Read the model definition and answer for the solid it produces. Units are mm, in the model's axes. A direction names the side the tool comes from. Give positions to 0.01 mm unless a question says otherwise; leave off trailing zeros. Order: outer loops, then holes, each group sorted by start corner. A loop starts at its lowest first (then second) coordinate and runs counter-clockwise, first axis right, second up. Notation, with made-up numbers: M 31,85.25 L 40,85.25 A21 ccw 40,115.25 Z; hole C 82,-32.75 d6. An arc over 180 degrees is marked long. One line per item, written item: value.
from build123d import *

# Parameters (mm, degrees)
SKETCH2_R           = 17.5
BOSS_EXTRUDE2_DEPTH = 30
SKETCH3_R           = 11.5
CUT_EXTRUDE1_DEPTH  = 30
CUT_EXTRUDE1_DRAFT  = -5
SKETCH4_R           = 15
SKETCH4_R_2         = 12.5
CUT_EXTRUDE2_DEPTH  = 5
SKETCH8_R           = 11.5
BOSS_EXTRUDE3_DEPTH = 30
SWEEP3_PITCH        = 10.666666667
SWEEP3_HEIGHT       = 24
SWEEP3_RADIUS       = 7.5
SKETCH10_R          = 3.5
SKETCH11_R          = 5
BOSS_EXTRUDE4_DEPTH = 50
SKETCH16_R          = 3.036795298
CUT_EXTRUDE7_DEPTH  = 6


with BuildPart() as part:
    # Sketch2 → Boss-Extrude2 (new body)
    with BuildSketch(Plane(origin=(0, 0, 0), x_dir=(1, 0, 0), z_dir=(0, 1, 0))):
        with Locations(Location((0, 0, 0), (0, 0, 270))):
            Circle(SKETCH2_R)
    extrude(amount=BOSS_EXTRUDE2_DEPTH)


with BuildPart() as cut_extrude1_tool:
    # Sketch3 → Cut-Extrude1 (with draft: the straight prism first)
    with BuildSketch(Plane.XZ):
        Circle(SKETCH3_R)
    extrude(amount=-CUT_EXTRUDE1_DEPTH)
    # Cut-Extrude1: the draft: its side faces are tilted about the plane it starts from
    cut_extrude1_sides = [cut_extrude1_tool.faces().sort_by_distance(p)[0] for p in [
        (-11.5, 15, 0),
    ]]
    draft(cut_extrude1_sides, Plane.XZ, CUT_EXTRUDE1_DRAFT)


with BuildPart() as part_1:
    add(part.part)

    # Cut-Extrude1: cut by cut_extrude1_tool
    add(cut_extrude1_tool.part, mode=Mode.SUBTRACT)

    # Sketch4 → Cut-Extrude2 (cut)
    with BuildSketch(Plane.XZ):
        with Locations(Location((0, 0.439504446, 0), (0, 0, 270))):
            Circle(SKETCH4_R)
        with Locations(Location((0, 0.439504446, 0), (0, 0, 270))):
            Circle(SKETCH4_R_2, mode=Mode.SUBTRACT)
    extrude(amount=-CUT_EXTRUDE2_DEPTH, mode=Mode.SUBTRACT)


with BuildPart() as body_2:
    # Sketch8 → Boss-Extrude3 (new body)
    with BuildSketch(Plane.XZ):
        with Locations(Location((0, 0, 0), (0, 0, 270))):
            Circle(SKETCH8_R)
    extrude(amount=BOSS_EXTRUDE3_DEPTH)


with BuildPart() as body_3:
    # Sweep3: sweep along a helix
    with BuildLine() as sweep3_path:
        Helix(SWEEP3_PITCH, SWEEP3_HEIGHT, SWEEP3_RADIUS, center=(0, 0, 0), direction=(0, -1, 0), lefthand=True)
    # Sketch10 → Sweep3 (sweep)
    with BuildSketch(Plane(origin=(0, 0, 0), x_dir=(0, 0, -1), z_dir=(1, 0, 0))):
        with Locations((-7.5, -16)):
            Circle(SKETCH10_R)
    sweep(path=sweep3_path.line, is_frenet=True)


with BuildPart() as body_2_1:
    add(body_2.part)

    # Combine1: cut body 3
    add(body_3.part, mode=Mode.SUBTRACT)

    # Sketch11 → Boss-Extrude4 (add)
    with BuildSketch(Plane.XZ.offset(30)):
        with Locations(Location((0, 0, 0), (0, 0, 270))):
            Circle(SKETCH11_R)
    extrude(amount=BOSS_EXTRUDE4_DEPTH)

    # Sketch16 → Cut-Extrude7 (cut)
    with BuildSketch(Plane.XZ.offset(30)):
        with Locations(Location((-7.743073418, -2.269070065, 0), (0, 0, 270))):
            Circle(SKETCH16_R)
    extrude(amount=-CUT_EXTRUDE7_DEPTH, mode=Mode.SUBTRACT)


solid = body_2_1.part
1) Which of the six approach directions +Z, -Z, +X, -X, +Y, -Y give full straight-line access (tool end or side, diameter ignored) to faces 1 (the face through (0, 0, 0)), 2 (the face through (-7.2, -23.8, 0))?
Reported:
face 1: +Z, -Z, +X, -X, +Y
face 2: none
2) Each of these flat-tipped pins is pushed along its axis until it touches: pin 1 Ø10 at (x, z) = (-8, 9) entering from -Y; pin 2 Ø2 at (x, y) = (-6.5, -22) entering from -Z; pin 3 Ø1.5 at (y, z) = (-52.5, -5) entering from -X; pin 4 Ø7 at (x, z) = (2, 5.5) entering from -Y. Where does it stop, or does it pass through?
Reported:
pin 1: stops at y = -30
pin 2: stops at z = -10.1
pin 3: stops at x = -2.63
pin 4: stops at y = -80
3) Find section C-C, the plane y = -28. Write down the section's boundary in (x, z).
Reported:
outline: C 0,0 d23; hole C -7.74,-2.27 d6.07
4) Determine the mould class of faces 3 (the face through (5.3, -30, 0.2)), 4 (the face through (-4.88, -54.65, 1.08)), 5 (the face through (0, -1, -7)), 6 (the face through (-10.708, -27.709, -1.611)) for opening direction X: +X half, -X half, draft (parallel to the pull), parting line (faces both ways), or undercut.
Reported:
face 3: draft
face 4: parting line
face 5: undercut
face 6: undercut
5) Consider probe 1 along Y at (x, z) = (7.5, 7.5); probe 2 along Y at (x, z) = (0.75, -9.5); probe 3 along X at (y, z) = (-26.5, -1). Determine where each line is inside the solid, lowest interval first.
Reported:
probe 1: y = -30 to -18.95, -15.72 to -8.28, -5.05 to 0
probe 2: y = -30 to -24.05, -18.35 to -13.38, -7.68 to 0
probe 3: x = -11.46 to -10.5, -4.98 to 11.46
6) Find section A-A, the plane y = -52. Write down the section's boundary in (x, z), plus the area to 3 significant figures.
Reported:
outline: C 0,0 d10
area: 78.5 mm^2
7) Find section B-B, the plane x = -3.25. Count the separate pieces of the cut face and the enclosed holes in it, plus the area to 3 significant figures.
Reported:
separate pieces: 1
enclosed holes: 4
area: 836 mm^2
